from build123d import *

# Parameters (mm, degrees)
BOSS_EXTRUDE1_DEPTH     = 9
FILLET1_R               = 2
CUT_EXTRUDE1_DEPTH      = 38.496666519
CUT_EXTRUDE1_DEPTH_BACK = 38.496666519
SKETCH3_R               = 2.5
BOSS_EXTRUDE2_DEPTH     = 10
CUT_EXTRUDE2_DEPTH      = 42.303752856
CUT_EXTRUDE2_DEPTH_BACK = 42.303752856
SKETCH4_R               = 0.75


with BuildPart() as part:
    # Sketch1 → Boss-Extrude1 (new, symmetric)
    with BuildSketch(Plane.XY):
        with BuildLine():
            ThreePointArc((-33.714795211, -0.491812162), (-34.647663561, 0.242423764), (-35, 1.376092494))
            Line((-35, 1.376092494), (-35, 10))
            Line((-35, 10), (35, 10))
            Line((35, 10), (35, 1.330500849))
            ThreePointArc((35, 1.330500849), (34.665188238, 0.222733667), (33.772851869, -0.514140034))
            Line((33.772851869, -0.514140034), (11.50283608, -9.844640883))
            ThreePointArc((11.50283608, -9.844640883), (11.12414042, -9.960775582), (10.729984211, -10))
            Line((10.729984211, -10), (-8.498371341, -10))
            ThreePointArc((-8.498371341, -10), (-8.861820571, -9.966698924), (-9.213166552, -9.867904657))
            Line((-9.213166552, -9.867904657), (-33.714795211, -0.491812162))
        make_face()
    extrude(amount=BOSS_EXTRUDE1_DEPTH, both=True)

    # Fillet1
    fillet1_edges = [part.edges().sort_by_distance(p)[0] for p in [
        (0, 10, -9),
        (0, 10, 9),
    ]]
    fillet(fillet1_edges, radius=FILLET1_R)

    # Sketch2 → Cut-Extrude1 (cut, two sides: drawn at the far end of the back side and taken through both)
    with BuildSketch(Plane(origin=(0, 0, 0), x_dir=(0, 0, -1), z_dir=(1, 0, 0)).offset(-CUT_EXTRUDE1_DEPTH_BACK)):
        with BuildLine():
            Line((-8, 8), (-8, -14.234256749))
            Line((-8, -14.234256749), (8, -14.234256749))
            Line((8, -14.234256749), (8, 1.330500849))
            Line((8, 1.330500849), (8, 8))
            ThreePointArc((8, 8), (7.707106781, 8.707106781), (7, 9))
            Line((7, 9), (-7, 9))
            ThreePointArc((-7, 9), (-7.707106781, 8.707106781), (-8, 8))
        make_face()
    extrude(amount=CUT_EXTRUDE1_DEPTH + CUT_EXTRUDE1_DEPTH_BACK, mode=Mode.SUBTRACT)

    # Sketch3 → Boss-Extrude2 (add)
    with BuildSketch(Plane(origin=(0, 10, 0), x_dir=(1, 0, 0), z_dir=(0, 1, 0))):
        with Locations(Location((0, 0, 0), (0, 0, 270))):
            Circle(SKETCH3_R)
    extrude(amount=BOSS_EXTRUDE2_DEPTH)

    # Sketch4 → Cut-Extrude2 (cut, two sides: drawn at the far end of the back side and taken through both)
    with BuildSketch(Plane.XY.offset(-CUT_EXTRUDE2_DEPTH_BACK)):
        with Locations((-30, 2)):
            Circle(SKETCH4_R)
        with Locations((-22, 2)):
            Circle(SKETCH4_R)
        with Locations((-5, -5)):
            Circle(SKETCH4_R)
        with Locations(Location((5, -5, 0), (0, 0, 180))):
            Circle(SKETCH4_R)
        with Locations(Location((22, 2, 0), (0, 0, 180))):
            Circle(SKETCH4_R)
        with Locations(Location((30, 2, 0), (0, 0, 180))):
            Circle(SKETCH4_R)
    extrude(amount=CUT_EXTRUDE2_DEPTH + CUT_EXTRUDE2_DEPTH_BACK, mode=Mode.SUBTRACT)


solid = part.part
Work out the finished part from the listing and answer in its coordinate system (mm). A direction names the side the tool comes from. Round coordinates to 2 decimals unless told otherwise and drop trailing zeros. Write each loop counter-clockwise with the first axis right and the second up, starting at its lowest first coordinate (ties: lowest second). Pieces come first, ordered by that corner, then holes.
1) Given pin 1 Ø1.5 at (x, z) = (-10, -1.5) entering from +Y; pin 2 Ø6 at (x, z) = (-7.5, -2.5) entering from -Y; pin 3 Ø6 at (x, y) = (11.5, 12.5) entering from +Z, each flat-ended and moving along its own axis, determine where each tip first touches the part or whether it passes through.
2) A tool of negligible diameter and unlimited length cuts with its end or side. For faces 1 (the flat face through (0, 1, 8)), 2 (the cylindrical face through (-34.64, 0.23, -8.49)), from which of +Z, -Z, +X, -X, +Y, -Y can it reach the whole face along a straight path? Write none if from no direction.
3) A cutting plane is placed at D-D (y = -5). Give the vertices of the cut face in (x, z), plus the area to 3 significant figures.
4) Straight lines are drawn through the part: line 1 (Z direction, x = -18, y = -0.25); line 2 (Y direction, x = -32, z = -5.5); line 3 (Y direction, x = 5, z = -8.35). For each, find the intervals that lie inside material, in ascending order.
5) The mould has two halves that part along Y. Classify faces 3 (the cylindrical face through (5.595, -4.544, 8.493)), 4 (the flat face through (0, 10, 3)), 5 (the cylindrical face through (-34.64, 0.23, 8.51)), 6 (the cylindrical face through (-22.75, 2.03, 8.49)): pulls with the +Y half, pulls with the -Y half, needs draft (parallel to the pull), parting line crosses it, or undercut.
6) A cutting plane is placed at B-B (y = 5.25). Give the vertices of the cut face in (x, z), plus the area to 3 significant figures.
7) A cutting plane is placed at C-C (z = -1.75). Give the vertices of the cut face in (x, y).
8) A cutting plane is placed at A-A (x = 5). Give the vertices of the cut face in (y, z).
Completed:
1. pin 1: stops at y = 10
1. pin 2: stops at y = 9
1. pin 3: stops at z = 8.32
2. face 1: +X, -X, -Y
2. face 2: +Z, -Z, -X, -Y
3. outline: (-21.93, -9) - (-5.75, -9) - (-5.75, -8) - (-21.93, -8) - close; (-21.93, 8) - (-5.75, 8) - (-5.75, 9) - (-21.93, 9) - close; (-4.25, -9) - (4.25, -9) - (4.25, -8) - (-4.25, -8) - close; (-4.25, 8) - (4.25, 8) - (4.25, 9) - (-4.25, 9) - close; (5.75, -9) - (23.07, -9) - (23.07, -8) - (5.75, -8) - close; (5.75, 8) - (23.07, 8) - (23.07, 9) - (5.75, 9) - close
3. area: 84.0 mm2
4. line 1: z = -9 to -8, 8 to 9
4. line 2: y = 9 to 10
4. line 3: y = -10 to -5.75, -4.25 to 9.48
5. face 3: undercut
5. face 4: pulls with the +Y half
5. face 5: pulls with the -Y half
5. face 6: undercut
6. outline: (-35, -9) - (35, -9) - (35, -8) - (-35, -8) - close; (-35, 8) - (35, 8) - (35, 9) - (-35, 9) - close
6. area: 140 mm2
7. outline: (-35, 9) - (35, 9) - (35, 10) - (1.79, 10) - (1.79, 20) - (-1.79, 20) - (-1.79, 10) - (-35, 10) - close
8. outline: (-10, -9) - (-5.75, -9) - (-5.75, -8) - (-10, -8) - close; (-10, 8) - (-5.75, 8) - (-5.75, 9) - (-10, 9) - close; (-4.25, -9) - (8, -9) arc R2 ccw to (10, -7) - (10, 7) arc R2 ccw to (8, 9) - (-4.25, 9) - (-4.25, 8) - (8, 8) arc R1 cw to (9, 7) - (9, -7) arc R1 cw to (8, -8) - (-4.25, -8) - close
